Design review of the part built by this model. Coordinates are the model's own, in mm. A direction names the side the tool comes from. Give positions to 0.01 mm unless a question says otherwise; leave off trailing zeros. Order: outer loops, then holes, each group sorted by start corner. A loop starts at its lowest first (then second) coordinate and runs counter-clockwise, first axis right, second up. Notation, with made-up numbers: (8, 44) -> (15, 44) arc R19 cw to (15, 65) -> close; hole circle Ø9 at (56, 21). An arc over 180 degrees is marked (long way). Use a Markdown table: item, result. Add a question column.
```python
from build123d import *

# Parameters (mm, degrees)
SKETCH2_R           = 25
BOSS_EXTRUDE1_DEPTH = 14.6
BOSS_EXTRUDE2_START = -40
SKETCH3_R           = 38.5
SKETCH3_R_2         = 25
BOSS_EXTRUDE2_DEPTH = 40
SKETCH4_W           = 14
SKETCH4_H           = 9
CUT_EXTRUDE1_DEPTH  = 45
MOVE_FACE1_BY       = 0.3
CHAMFER3_SIZE       = 1.5
CHAMFER4_SIZE       = 3


with BuildPart() as part:
    # Sketch2 → Boss-Extrude1 (new body)
    with BuildSketch(Plane.XY):
        with BuildLine():
            ThreePointArc((53.163386549, 25.920934205), (52.371116098, 27.486482097), (51.532756355, 29.027840461))
            ThreePointArc((51.532756355, 29.027840461), (46.843166468, 28.705871605), (42.269756881, 27.619666278))
            ThreePointArc((42.269756881, 27.619666278), (33.778781557, 29.925389145), (32.513343984, 38.632379879))
            ThreePointArc((32.513343984, 38.632379879), (34.14289326, 43.041516576), (35.027782197, 47.658105016))
            ThreePointArc((35.027782197, 47.658105016), (33.598715171, 48.676142393), (32.140079536, 49.651342246))
            ThreePointArc((32.140079536, 49.651342246), (28.137280301, 47.186891894), (24.59251201, 44.099735432))
            ThreePointArc((24.59251201, 44.099735432), (16.002603901, 42.195398652), (10.835774224, 49.316977899))
            ThreePointArc((10.835774224, 49.316977899), (10.229640458, 53.978363864), (8.867735075, 58.47737831))
            ThreePointArc((8.867735075, 58.47737831), (7.129253506, 58.714685078), (5.384497826, 58.900319885))
            ThreePointArc((5.384497826, 58.900319885), (2.985482308, 54.857963913), (1.281419009, 50.477086658))
            ThreePointArc((1.281419009, 50.477086658), (-5.439577457, 44.798950837), (-13.324140826, 48.703650616))
            ThreePointArc((-13.324140826, 48.703650616), (-16.027099693, 52.549418501), (-19.323803285, 55.900188962))
            ThreePointArc((-19.323803285, 55.900188962), (-20.973434219, 55.302401001), (-22.604607447, 54.655944065))
            ThreePointArc((-22.604607447, 54.655944065), (-22.850253703, 49.96173751), (-22.323231644, 45.290745645))
            ThreePointArc((-22.323231644, 45.290745645), (-25.635617173, 37.139603271), (-34.431655785, 36.93290392))
            ThreePointArc((-34.431655785, 36.93290392), (-38.612224452, 39.082034648), (-43.08849119, 40.516939993))
            ThreePointArc((-43.08849119, 40.516939993), (-44.271360923, 39.22100332), (-45.415269568, 37.890550135))
            ThreePointArc((-45.415269568, 37.890550135), (-43.451271965, 33.619879148), (-40.813898952, 29.728840617))
            ThreePointArc((-40.813898952, 29.728840617), (-39.958845938, 20.972020177), (-47.651293351, 16.701274026))
            ThreePointArc((-47.651293351, 16.701274026), (-52.351753916, 16.661427647), (-56.982125035, 15.851748354))
            ThreePointArc((-56.982125035, 15.851748354), (-57.427252367, 14.154546443), (-57.821840745, 12.444887799))
            ThreePointArc((-57.821840745, 12.444887799), (-54.098127465, 9.576111636), (-49.95459387, 7.356416476))
            ThreePointArc((-49.95459387, 7.356416476), (-45.127984655, 0), (-49.95459387, -7.356416476))
            ThreePointArc((-49.95459387, -7.356416476), (-54.098127465, -9.576111636), (-57.821840745, -12.444887799))
            ThreePointArc((-57.821840745, -12.444887799), (-57.427252367, -14.154546443), (-56.982125035, -15.851748354))
            ThreePointArc((-56.982125035, -15.851748354), (-52.351753916, -16.661427647), (-47.651293351, -16.701274026))
            ThreePointArc((-47.651293351, -16.701274026), (-39.958845938, -20.972020177), (-40.813898952, -29.728840617))
            ThreePointArc((-40.813898952, -29.728840617), (-43.451271965, -33.619879148), (-45.415269568, -37.890550135))
            ThreePointArc((-45.415269568, -37.890550135), (-44.271360923, -39.22100332), (-43.08849119, -40.516939993))
            ThreePointArc((-43.08849119, -40.516939993), (-38.612224452, -39.082034648), (-34.431655785, -36.93290392))
            ThreePointArc((-34.431655785, -36.93290392), (-25.635617173, -37.139603271), (-22.323231644, -45.290745645))
            ThreePointArc((-22.323231644, -45.290745645), (-22.850253703, -49.96173751), (-22.604607446, -54.655944065))
            ThreePointArc((-22.604607446, -54.655944065), (-20.973434219, -55.302401001), (-19.323803285, -55.900188962))
            ThreePointArc((-19.323803285, -55.900188962), (-16.027099693, -52.549418501), (-13.324140826, -48.703650616))
            ThreePointArc((-13.324140826, -48.703650616), (-5.439577457, -44.798950837), (1.281419009, -50.477086658))
            ThreePointArc((1.281419009, -50.477086658), (2.985482308, -54.857963913), (5.384497826, -58.900319885))
            ThreePointArc((5.384497826, -58.900319885), (7.129253506, -58.714685078), (8.867735075, -58.47737831))
            ThreePointArc((8.867735075, -58.47737831), (10.229640457, -53.978363864), (10.835774224, -49.316977899))
            ThreePointArc((10.835774224, -49.316977899), (16.002603901, -42.195398652), (24.59251201, -44.099735432))
            ThreePointArc((24.59251201, -44.099735432), (28.137280301, -47.186891894), (32.140079536, -49.651342246))
            ThreePointArc((32.140079536, -49.651342246), (33.598715171, -48.676142393), (35.027782197, -47.658105016))
            ThreePointArc((35.027782197, -47.658105016), (34.14289326, -43.041516576), (32.513343984, -38.632379879))
            ThreePointArc((32.513343984, -38.632379879), (33.778781557, -29.925389145), (42.269756881, -27.619666278))
            ThreePointArc((42.269756881, -27.619666278), (46.843166468, -28.705871605), (51.532756355, -29.027840461))
            ThreePointArc((51.532756355, -29.027840461), (52.371116098, -27.486482097), (53.163386549, -25.920934206))
            ThreePointArc((53.163386549, -25.920934206), (50.234420683, -22.244376547), (46.742498465, -19.097569199))
            ThreePointArc((46.742498465, -19.097569199), (43.816647437, -10.799833626), (50.263509857, -4.812264433))
            ThreePointArc((50.263509857, -4.812264433), (54.817847718, -3.648682075), (59.11989973, -1.754410251))
            ThreePointArc((59.11989973, -1.754410251), (59.145925468, 0), (59.11989973, 1.754410251))
            ThreePointArc((59.11989973, 1.754410251), (54.817847718, 3.648682075), (50.263509857, 4.812264433))
            ThreePointArc((50.263509857, 4.812264433), (43.816647437, 10.799833626), (46.742498465, 19.097569199))
            ThreePointArc((46.742498465, 19.097569199), (50.234420683, 22.244376547), (53.163386549, 25.920934205))
        make_face()
        Circle(SKETCH2_R, mode=Mode.SUBTRACT)
    extrude(amount=BOSS_EXTRUDE1_DEPTH)

    # Sketch3 → Boss-Extrude2 (add)
    with BuildSketch(Plane.XY.offset(14.6).offset(BOSS_EXTRUDE2_START)):
        Circle(SKETCH3_R)
        Circle(SKETCH3_R_2, mode=Mode.SUBTRACT)
    extrude(amount=BOSS_EXTRUDE2_DEPTH)

    # Sketch4 → Cut-Extrude1 (cut)
    with BuildSketch(Plane.XY.offset(14.6)):
        with Locations((0, 25)):
            Rectangle(SKETCH4_W, SKETCH4_H)
    extrude(amount=-CUT_EXTRUDE1_DEPTH, mode=Mode.SUBTRACT)

    # Move Face1: a face moved inward by 0.3
    extrude(part.faces().sort_by_distance((0, 29.5, -5.4))[0], amount=MOVE_FACE1_BY, dir=(0, 1, 0), mode=Mode.SUBTRACT)

    # Chamfer3
    chamfer3_edges = [part.edges().sort_by_distance(p)[0] for p in [
        (-38.5, 0, -25.4),
        (0, -25, -25.4),
        (0, -25, 14.6),
    ]]
    chamfer(chamfer3_edges, length=CHAMFER3_SIZE)

    # Chamfer4
    chamfer4_edges = [part.edges().sort_by_distance(p)[0] for p in [
        (-38.5, 0, 0),
    ]]
    chamfer(chamfer4_edges, length=CHAMFER4_SIZE)


solid = part.part
```
1) Insertion check: pin 1 (8 mm diameter, centred on x = -8.5, y = -19.5, fed in from -Z); pin 2 (3 mm diameter, centred on y = 25.5, z = -2, fed in from +X); pin 3 (1 mm diameter, centred on x = 22, z = 8.5, fed in from -Y). Each pin has a flat end and moves straight along its axis. Give the tip position at first contact, or say it passes through.
2) Machinability: for faces 1 (the cylindrical face through (34.16, -43.11, 7.2)), 2 (the cylindrical face through (3.014, 54.917, 7.198)), 3 (the cylindrical face through (2.957, -54.799, 7.198)), 4 (the cylindrical face through (-20.95, 55.31, 7.2)), which of the approach directions +Z, -Z, +X, -X, +Y, -Y give a long, thin tool a straight path to every point of the face, cutting with its end or side? Answer none if there is none.
3) For L1, parallel to Y at x = 0, z = -10; L2, parallel to X at y = 0, z = -6; L3, parallel to Y at x = 53, z = 0.5, list the stretches that pass through material, from the lowest coordinate up. Write a range as [from, to].
4) Add section A-A (z = -7). Give the boundary of the cut face in (x, y), then the cut area to 3 significant figures.
5) The part is to be moulded in two halves that separate along X. For faces 5 (the cylindrical face through (52.383, 27.465, 7.198)), 6 (the conical face through (-1.02, -25.22, 13.34)), 7 (the flat face through (-17, -39, 0)), say which applies: +X half, -X half, draft (parallel to the pull), parting line (faces both ways), or undercut.
Worked answers:
| question | item | result |
|---|---|---|
| 1 | pin 1 | z = -24.17 |
| 1 | pin 2 | x = 32.44 |
| 1 | pin 3 | y = -42.55 |
| 2 | face 1 | +Z, -Z, +X |
| 2 | face 2 | +Z, -Z, +Y |
| 2 | face 3 | +Z, -Z, -Y |
| 2 | face 4 | +Z, -Z, -X, +Y |
| 3 | L1 | [-38.5, -25], [29.8, 38.5] |
| 3 | L2 | [-38.5, -25], [25, 38.5] |
| 3 | L3 | [-26.25, -25.68], [-4.21, 4.21], [25.68, 26.25] |
| 4 | outline | circle Ø77 at (0, 0); hole (-7, 24) arc R25 ccw (long way) to (7, 24) -> (7, 29.8) -> (-7, 29.8) -> close |
| 4 | area | 2,620 mm^2 |
| 5 | face 5 | +X half |
| 5 | face 6 | undercut |
| 5 | face 7 | draft |
